Answer from the drawing. Dimensions are ordinates in mm from the lowest x, y and z of the part. Give positions to 0.01 mm unless a question says otherwise; leave off trailing zeros. Loops run counter-clockwise (first coordinate to the right, second up) from the corner with the lowest first, then second, coordinate; pieces in that order, holes last.
Item 1: Section C-C, the plane z = 88 is taken. Give the vertices of the cut face in (x, y), and give its area (3 significant figures).
Item 2: Section A-A, the plane z = 55 is taken. Give the vertices of the cut face in (x, y).
Item 3: Section D-D, the plane y = 15 is taken. Give the vertices of the cut face in (x, z), and give its area (3 significant figures).
Item 4: Consider line 1 along Z through (x, y) = (55, 22.25); line 2 along Z through (x, y) = (55, 4.75); line 3 along X through (y, z) = (20, 29). Determine where each line is inside the solid, lowest interval first.
Item 5: Section B-B, the plane x = 55 is taken. Give the vertices of the cut face in (y, z), and give its area (3 significant figures).
Item 6: Each of these flat-tipped pins is pushed along its axis until it touches: pin 1 Ø7 at (x, y) = (55, 15) entering from +Z; pin 2 Ø12 at (x, z) = (42.5, 55) entering from -Y; pin 3 Ø4 at (y, z) = (13, 23.5) entering from -X; pin 4 Ø21 at (x, z) = (55, 55) entering from +Y. Where does it stop, or does it pass through?
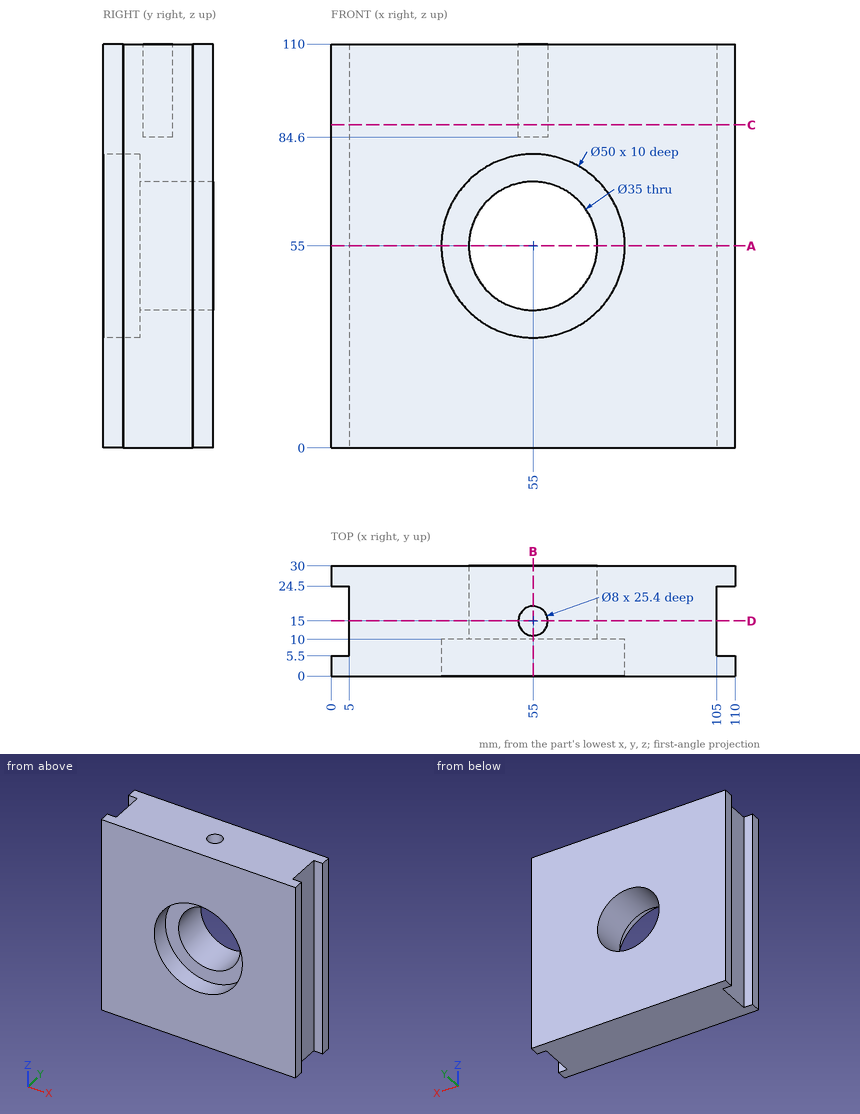
Worked answers:
1. outline: (0, 0) - (110, 0) - (110, 5.5) - (105, 5.5) - (105, 24.5) - (110, 24.5) - (110, 30) - (0, 30) - (0, 24.5) - (5, 24.5) - (5, 5.5) - (0, 5.5) - close; hole circle Ø8 at (55, 15)
1. area: 3,060 mm2
2. outline: (0, 0) - (30, 0) - (30, 10) - (37.5, 10) - (37.5, 30) - (0, 30) - (0, 24.5) - (5, 24.5) - (5, 5.5) - (0, 5.5) - close; (72.5, 10) - (80, 10) - (80, 0) - (110, 0) - (110, 5.5) - (105, 5.5) - (105, 24.5) - (110, 24.5) - (110, 30) - (72.5, 30) - close
3. outline: (5, 0) - (105, 0) - (105, 110) - (59, 110) - (59, 84.6) - (51, 84.6) - (51, 110) - (5, 110) - close; hole circle Ø35 at (55, 55)
3. area: 9,830 mm2
4. line 1: z = 0 to 37.5, 72.5 to 110
4. line 2: z = 0 to 30, 80 to 110
4. line 3: x = 5 to 105
5. outline: (0, 0) - (30, 0) - (30, 37.5) - (10, 37.5) - (10, 30) - (0, 30) - close; (0, 80) - (10, 80) - (10, 72.5) - (30, 72.5) - (30, 110) - (19, 110) - (19, 84.6) - (11, 84.6) - (11, 110) - (0, 110) - close
5. area: 1,900 mm2
6. pin 1: stops at z = 84.6
6. pin 2: stops at y = 10
6. pin 3: stops at x = 5
6. pin 4: passes through
